Autodesk Inventor part; units mm, degrees
ref_plane "Work Plane1" through (0, -15, 0) normal (0, -1, 0) x (1, 0, 0)
ref_plane "Work Plane2" through (0, -15, 0) normal (0, -1, 0) x (1, 0, 0)
ref_plane "YZ Plane" through (0, 0, 0) normal (1, 0, 0) x (0, 1, 0)
sketch "Sketch1" plane through (0, 0, 0) normal (0, 1, 0) x (-1, 0, 0)
  line L0 (0, -20) -> (40, -20)
  line L1 (40, -20) -> (40, -38)
  line L2 (0, -20) -> (0, 0)
  line L3 (0, 0) -> (2.5, 0)
  line L4 (2.5, 0) -> (2.5, 3)
  line L5 (2.5, 3) -> (-10, 3)
  line L6 (-10, 3) -> (-10, -38)
  line L7 (-10, -38) -> (40, -38)
  circle A0 centre (0, -28) radius 4
  point P0 (-3.75, 3)
  point P1 (1.25, 0)
  dimension "d1" = 40
  dimension "d2" = 18
  dimension "d4" = 12.5
  dimension "d5" = 10
  dimension "d6" = 3
  dimension "d7" = 20
  dimension "d8" = 8
  dimension "d9" = 10
  dimension "d10" = 10
extrude "Extrusion1" add sketch "Sketch1" along normal blind 20
sketch "Sketch2" plane through (0, 0, 0) normal (0, -1, 0) x (1, 0, 0)
  point P0 (0, 0)
sketch "Sketch3" plane through (0, 0, 0) normal (0, -1, 0) x (1, 0, 0)
  line L0 (10, -38) -> (-40, -38)
  line L1 (-8, -38) -> (-8, -20)
  line L2 (-40, -20) -> (0, -20)
  line L3 (10, 3) -> (10, -38)
  line L4 (-8, -38) -> (-40, -38)
  line L5 (-40, -38) -> (-40, -20)
  line L6 (-40, -20) -> (-8, -20)
  point P0 (0, 0)
  dimension "d13" = 18
extrude "Extrusion2" add sketch "Sketch3" along normal blind 15
ref_plane "Work Plane1" through (0, -15, 0) normal (0, -1, 0) x (1, 0, 0)
mirror "Mirror1" about plane through (0, -15, 0) normal (0, -1, 0) of "Extrusion1"
ref_plane "Work Plane2" through (0, -15, 0) normal (0, -1, 0) x (1, 0, 0)
mirror "Mirror2" about plane through (0, -15, 0) normal (0, -1, 0) of "Extrusion2"
sketch "Sketch4" plane through (10, 20, -38) normal (0, 0, -1) x (-1, 0, 0)
  circle A0 centre (25, -12.5) radius 7.5
  circle A1 centre (25, -57.5) radius 7.5
  line L0 (50, -70) -> (50, 0)
  line L1 (0, 0) -> (50, 0)
  line L2 (0, -70) -> (50, -70)
  point P0 (10, -20)
  dimension "d18" = 15
  dimension "d19" = 15
  dimension "d20" = 25
  dimension "d21" = 12.5
  dimension "d22" = 12.5
  dimension "d23" = 25
hole "Hole1" at (-15, 7.5, -38) at (-15, -37.5, -38) direction (0, 0, 1) diameter 15 depth 8 tip angle 118
sketch "Sketch5" plane through (10, 20, -38) normal (0, 0, -1) x (-1, 0, 0)
  circle A0 centre (25, -12.5) radius 4.2
  circle A1 centre (25, -57.5) radius 4.2
  line L0 (50, -70) -> (50, 0)
  line L1 (0, 0) -> (50, 0)
  line L2 (0, -70) -> (50, -70)
  point P0 (10, -20)
  dimension "d31" = 8.4
  dimension "d32" = 8.4
  dimension "d33" = 25
  dimension "d34" = 12.5
  dimension "d35" = 25
  dimension "d36" = 12.5
hole "Hole2" at (-15, 7.5, -38) at (-15, -37.5, -38) direction (0, 0, 1) diameter 8.4 end through all
chamfer "Chamfer1" distance 2 angle 45 1 edges at (-15, 20, -38) measured on face at (-33.7241, -8.9202, -38)
chamfer "Chamfer2" distance 2 angle 45 1 edges at (-40, -16, -38) measured on face at (-33.7241, -21.7465, -38)
chamfer "Chamfer3" distance 2 angle 45 1 edges at (-14, -50, -38) measured on face at (-32.3908, -21.7465, -38)
chamfer "Chamfer4" distance 2 angle 45 1 edges at (10, 9, -38) measured on face at (-32.3908, -21.0798, -38)
chamfer "Chamfer5" distance 2 angle 45 1 edges at (10, -39, -38) measured on face at (-32.3908, -21.0798, -38)
chamfer "Chamfer6" distance 2 angle 45 1 edges at (10, 20, -16.5) measured on face at (-28, 20, -28)
chamfer "Chamfer7" distance 2 angle 45 1 edges at (10, -50, -16.5) measured on face at (-28, -50, -28)
properties part number "Lager" material "Iron, Cast"
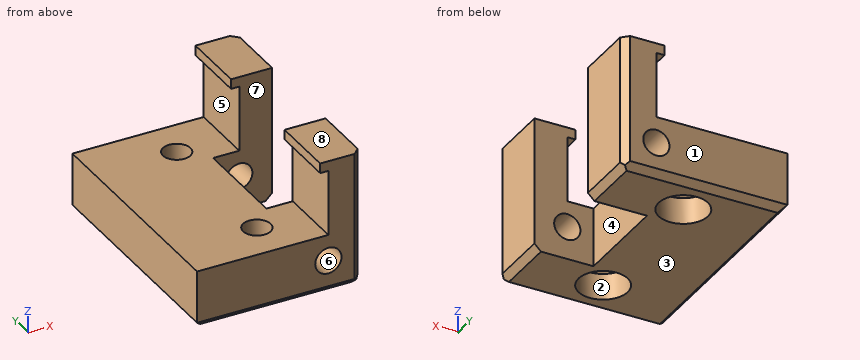
Could you check a few things on this model? Use its own coordinates, in mm. Face numbers are marked on the shaded views. A direction names the side the tool comes from. Coordinates: 2 decimals unless noted, no trailing zeros. Loops run counter-clockwise (first coordinate to the right, second up) from the corner with the lowest first, then second, coordinate; pieces in that order, holes last.
1. Imagine slicing it at C-C (z = -11). Please give me the cut outline in (x, y).
2. Imagine slicing it at A-A (x = -15). Please give me the cut outline in (y, z), and give its area (3 significant figures).
3. Imagine slicing it at B-B (y = -37.5). Please give me the cut outline in (x, z), and give its area (3 significant figures).
4. We'd pull the mould along Z, two halves only. Please class the marked faces 6, 7 and 8: released by +Z, released by -Z, zero draft, split by the parting line, or undercut.
5. For the marked faces 1, 2, 3, 4 and 5, which set-ups out of +Z, -Z, +X, -X, +Y, -Y let a thin tool reach every point of the face, with its end or its side?
6. Imagine slicing it at D-D (x = 1). Please give me the cut outline in (y, z), and give its area (3 significant figures).
7. I need wall thicknesses on L1, parallel to Y at x = -15, z = -22; L2, parallel to Y at x = -15, z = -33.5; L3, parallel to Y at x = 6.5, z = 0.5. Which ranges of each line are inside material? Lowest first, please.
8. For P1, Ø19.5, axis at x = -15, y = -37.5, coming from the +Z side; P2, Ø8, axis at y = -18, z = -26, coming from the +X side; P3, Ø22, axis at y = -35.5, z = -8, coming from the -X side, each with a flat end and sliding along its axis, tell me the tip position at first contact or that it passes through.
Computed values:
1. outline: (0, -50) - (8, -50) - (10, -48) - (10, -30) - (0, -30) - close; (0, 0) - (10, 0) - (10, 18) - (8, 20) - (0, 20) - close
2. outline: (-50, -36) - (-48, -38) - (-45, -38) - (-45, -30) - (-41.7, -28.02) - (-41.7, -20) - (-50, -20) - close; (-33.3, -28.02) - (-30, -30) - (-30, -38) - (0, -38) - (0, -30) - (3.3, -28.02) - (3.3, -20) - (-33.3, -20) - close; (11.7, -28.02) - (15, -30) - (15, -38) - (18, -38) - (20, -36) - (20, -20) - (11.7, -20) - close
2. area: 835 mm2
3. outline: (-40, -36) - (-38, -38) - (-22.5, -38) - (-22.5, -30) - (-19.2, -28.02) - (-19.2, -20) - (-40, -20) - close; (-10.8, -28.02) - (-7.5, -30) - (-7.5, -38) - (8, -38) - (10, -36) - (10, 3) - (-2.5, 3) - (-2.5, 0) - (0, 0) - (0, -20) - (-10.8, -20) - close; hole circle Ø8 at (0, -28)
3. area: 873 mm2
4. face 6: undercut
4. face 7: zero draft
4. face 8: released by +Z
5. face 1: +Z, -Z, +X, -X, +Y
5. face 2: -Z
5. face 3: -Z, +X, -X, +Y, -Y
5. face 4: +Z, -Z, +X
5. face 5: -X, +Y, -Y
6. outline: (-50, -36) - (-48, -38) - (-30, -38) - (-30, -31.87) - (-50, -31.87) - close; (-50, -24.13) - (-30, -24.13) - (-30, 3) - (-50, 3) - close; (0, -38) - (18, -38) - (20, -36) - (20, -31.87) - (0, -31.87) - close; (0, -24.13) - (20, -24.13) - (20, 3) - (0, 3) - close
6. area: 1,330 mm2
7. L1: y = -50 to -41.7, -33.3 to 3.3, 11.7 to 20
7. L2: y = -50 to -45, -30 to 0, 15 to 20
7. L3: y = -50 to -30, 0 to 20
8. P1: stops at z = -20
8. P2: stops at x = -8
8. P3: stops at x = -2.5
